from build123d import *

# Parameters (mm, degrees)
SKETCH1_W           = 29.8
SKETCH1_H           = 30.1
BOSS_EXTRUDE1_DEPTH = 9.9
CUT_EXTRUDE1_DEPTH  = 8.1
SKETCH3_R           = 2.8
CUT_EXTRUDE2_DEPTH  = 44.123775345


with BuildPart() as part:
    # Sketch1 → Boss-Extrude1 (new body)
    with BuildSketch(Plane.XY):
        with Locations((14.9, 15.05)):
            Rectangle(SKETCH1_W, SKETCH1_H)
    extrude(amount=BOSS_EXTRUDE1_DEPTH)

    # Sketch2 → Cut-Extrude1 (cut)
    with BuildSketch(Plane.XY.offset(9.9)):
        Polygon((7.8, 30.1), (7.8, 28.466915374), (17.8, 28.466915374), (17.8, 13.966915374), (1.8, 13.966915374), (1.8, 28.466915374), (1.8, 30.1), align=None)
    extrude(amount=-CUT_EXTRUDE1_DEPTH, mode=Mode.SUBTRACT)

    # Sketch3 → Cut-Extrude2 (cut, through all)
    with BuildSketch(Plane.XY.offset(1.8)):
        with Locations((14.3, 17.466915374)):
            Circle(SKETCH3_R)
    extrude(amount=-CUT_EXTRUDE2_DEPTH, mode=Mode.SUBTRACT)


solid = part.part
Verification items for the finished model (mm, model axes). A direction names the side the tool comes from. Round coordinates to 2 decimals unless told otherwise and drop trailing zeros. Loops run counter-clockwise (first coordinate to the right, second up) from the corner with the lowest first, then second, coordinate; pieces in that order, holes last. Notation, with made-up numbers: (82, 23) - (136, 23) arc R4 cw to (136, 28) - close; hole circle Ø4 at (65, 43). An arc over 180 degrees is marked (long way). Use a Markdown table: item, result. Add a question column.
1. Section check A-A, the plane x = 14.3. Record the boundary of the cut face in (y, z), plus the area to 3 significant figures.
2. Gauge pin test, flat ends, axial feed: pin 1 (3.5 mm diameter, centred on x = 14.3, y = 17.47, fed in from -Z); pin 2 (2 mm diameter, centred on x = 9, y = 20, fed in from +Z). Record the tip position at first contact, or that the pin passes through.
3. Thickness scan on probe 1 along Y at (x, z) = (14.3, 0.55); probe 2 along Y at (x, z) = (15.75, 3); probe 3 along Z at (x, y) = (17.25, 27). Record the ranges inside material, lowest first. Write a range as [from, to].
4. Section check D-D, the plane x = 9.5. Record the boundary of the cut face in (y, z), plus the area to 3 significant figures.
5. Access from +Z, -Z, +X, -X, +Y, -Y to the whole of each face (thin tool, end or side, straight path). Record for faces 5 (the face through (1.8, 22, 6)), 6 (the face through (15, 12, 9.9)), 7 (the face through (13, 28.467, 6)).
6. Release check for a two-part mould opening along Y. For faces 1 (the face through (10, 22, 1.8)), 2 (the face through (29.8, 15, 5)), 3 (the face through (15, 30.1, 5)), 4 (the face through (15, 0, 5)) record: released by +Y, released by -Y, zero draft, split by the parting line, or undercut.
7. Section check C-C, the plane y = 16. Record the boundary of the cut face in (x, z).
8. Section check B-B, the plane z = 2.75. Record the boundary of the cut face in (x, y), plus the area to 3 significant figures.
Checks:
| question | item | result |
|---|---|---|
| 1 | outline | (0, 0) - (14.67, 0) - (14.67, 1.8) - (13.97, 1.8) - (13.97, 9.9) - (0, 9.9) - close; (20.27, 0) - (30.1, 0) - (30.1, 9.9) - (28.47, 9.9) - (28.47, 1.8) - (20.27, 1.8) - close |
| 1 | area | 170 mm^2 |
| 2 | pin 1 | passes through |
| 2 | pin 2 | stops at z = 1.8 |
| 3 | probe 1 | y = [0, 14.67], [20.27, 30.1] |
| 3 | probe 2 | y = [0, 13.97], [28.47, 30.1] |
| 3 | probe 3 | z = [0, 1.8] |
| 4 | outline | (0, 0) - (30.1, 0) - (30.1, 9.9) - (28.47, 9.9) - (28.47, 1.8) - (13.97, 1.8) - (13.97, 9.9) - (0, 9.9) - close |
| 4 | area | 181 mm^2 |
| 5 | face 5 | +Z, +Y |
| 5 | face 6 | +Z, +X, -X, +Y, -Y |
| 5 | face 7 | +Z |
| 6 | face 1 | undercut |
| 6 | face 2 | zero draft |
| 6 | face 3 | released by +Y |
| 6 | face 4 | released by -Y |
| 7 | outline | (0, 0) - (11.92, 0) - (11.92, 1.8) - (1.8, 1.8) - (1.8, 9.9) - (0, 9.9) - close; (16.68, 0) - (29.8, 0) - (29.8, 9.9) - (17.8, 9.9) - (17.8, 1.8) - (16.68, 1.8) - close |
| 8 | outline | (0, 0) - (29.8, 0) - (29.8, 30.1) - (7.8, 30.1) - (7.8, 28.47) - (17.8, 28.47) - (17.8, 13.97) - (1.8, 13.97) - (1.8, 30.1) - (0, 30.1) - close |
| 8 | area | 655 mm^2 |
